Here's how the part is built. I have some questions about the finished solid (model axes, mm). A direction names the side the tool comes from. Round coordinates to 2 decimals unless told otherwise and drop trailing zeros. Order: outer loops, then holes, each group sorted by start corner. A loop starts at its lowest first (then second) coordinate and runs counter-clockwise, first axis right, second up.
```python
from build123d import *

# Parameters (mm, degrees)
SKETCH1_R           = 10.5
SKETCH1_R_2         = 1.85
BOSS_EXTRUDE1_DEPTH = 6
SKETCH2_R           = 5.25
CUT_EXTRUDE1_DEPTH  = 5
SKETCH3_R           = 2.8
CUT_EXTRUDE2_DEPTH  = 2
SKETCH5_R           = 2.85
SKETCH5_R_2         = 1.85
CUT_EXTRUDE4_DEPTH  = 3


with BuildPart() as part:
    # Sketch1 → Boss-Extrude1 (new body)
    with BuildSketch(Plane.XY):
        Circle(SKETCH1_R)
        with Locations((7, 0)):
            Circle(SKETCH1_R_2, mode=Mode.SUBTRACT)
        with Locations((0, -7)):
            Circle(SKETCH1_R_2, mode=Mode.SUBTRACT)
        with Locations((-7, 0)):
            Circle(SKETCH1_R_2, mode=Mode.SUBTRACT)
        with Locations((0, 7)):
            Circle(SKETCH1_R_2, mode=Mode.SUBTRACT)
    extrude(amount=BOSS_EXTRUDE1_DEPTH)

    # Sketch2 → Cut-Extrude1 (cut)
    with BuildSketch(Plane(origin=(0, 0, 0), x_dir=(-1, 0, 0), z_dir=(0, 0, -1))):
        Circle(SKETCH2_R)
    extrude(amount=-CUT_EXTRUDE1_DEPTH, mode=Mode.SUBTRACT)

    # Sketch3 → Cut-Extrude2 (cut, through all)
    with BuildSketch(Plane(origin=(0, 0, 5), x_dir=(-1, 0, 0), z_dir=(0, 0, -1))):
        Circle(SKETCH3_R)
    extrude(amount=-CUT_EXTRUDE2_DEPTH, mode=Mode.SUBTRACT)

    # Sketch5 → Cut-Extrude4 (cut)
    with BuildSketch(Plane(origin=(0, 0, 6), x_dir=(-1, 0, 0), z_dir=(0, 0, -1))):
        with Locations((0, 7)):
            Circle(SKETCH5_R)
        with Locations((0, 7)):
            Circle(SKETCH5_R_2, mode=Mode.SUBTRACT)
        with Locations((7, 0)):
            Circle(SKETCH5_R)
        with Locations((0, -7)):
            Circle(SKETCH5_R)
        with Locations((-7, 0)):
            Circle(SKETCH5_R)
        with Locations((-7, 0)):
            Circle(SKETCH5_R_2, mode=Mode.SUBTRACT)
    extrude(amount=CUT_EXTRUDE4_DEPTH, mode=Mode.SUBTRACT)


solid = part.part
```
1) If we section it at D-D (x = -2.5): Write out the boundary of the cut face in (y, z).
2) I'm going to push flat-ended pins straight in: pin 1 (2.5 mm diameter, centred on x = 0.5, y = -7.5, fed in from +Z); pin 2 (6.5 mm diameter, centred on x = 0, y = -7, fed in from -Z); pin 3 (3 mm diameter, centred on y = -7.5, z = 1.5, fed in from -X); pin 4 (1 mm diameter, centred on x = 6, z = 1, fed in from +Y). Where does each tip first touch, or does it pass through?
3) For faces 4 (the flat face through (9.1, 0, 3)), 5 (the cylindrical face through (-8.85, 0.07, 1.48)), 6 (the cylindrical face through (3.676, 3.748, 1.909)), which set-ups out of +Z, -Z, +X, -X, +Y, -Y let a thin tool reach every point of the face, with its end or its side?
4) If we section it at C-C (z = 1.1): Write out the boundary of the cut face in (x, y).
5) We'd pull the mould along X, two halves only. Please class faces 1 (the cylindrical face through (10, 3.2, 3)), 2 (the flat face through (2.2, -2.2, 6)), 3 (the cylindrical face through (-9.718, 0.856, 4.521)): +X half, -X half, draft (parallel to the pull), parting line (faces both ways), or undercut.
6) If we section it at A-A (x = 0): Write out the boundary of the cut face in (y, z).
7) If we section it at B-B (y = -6.5): Write out the boundary of the cut face in (x, z).
8) I need wall thicknesses on line 1 (Y direction, x = -2.5, z = 4.5); line 2 (Y direction, x = 0, z = 4.1); line 3 (Y direction, x = 0, z = 1.2). Which ranges of each line are inside material? Lowest first, please.
Solutions:
1. outline: (-10.2, 0) - (-4.62, 0) - (-4.62, 5) - (-1.26, 5) - (-1.26, 6) - (-5.63, 6) - (-5.63, 3) - (-8.37, 3) - (-8.37, 6) - (-10.2, 6) - close; (1.26, 5) - (4.62, 5) - (4.62, 0) - (10.2, 0) - (10.2, 6) - (8.37, 6) - (8.37, 3) - (5.63, 3) - (5.63, 6) - (1.26, 6) - close
2. pin 1: stops at z = 3
2. pin 2: stops at z = 0
2. pin 3: stops at x = -8.62
2. pin 4: stops at y = 8.94
3. face 4: +Z
3. face 5: +Z, -Z
3. face 6: -Z
4. outline: circle Ø21 at (0, 0); hole (-5.22, -0.52) arc R5.25 ccw to (-0.52, -5.22) arc R1.85 ccw (long way) to (0.52, -5.22) arc R5.25 ccw to (5.22, -0.52) arc R1.85 ccw (long way) to (5.22, 0.52) arc R5.25 ccw to (0.52, 5.22) arc R1.85 ccw (long way) to (-0.52, 5.22) arc R5.25 ccw to (-5.22, 0.52) arc R1.85 ccw (long way) to start
5. face 1: parting line
5. face 2: draft
5. face 3: undercut
6. outline: (-10.5, 0) - (-8.85, 0) - (-8.85, 3) - (-9.85, 3) - (-9.85, 6) - (-10.5, 6) - close; (-4.15, 5) - (-2.8, 5) - (-2.8, 6) - (-4.15, 6) - close; (2.8, 5) - (4.15, 5) - (4.15, 6) - (2.8, 6) - close; (8.85, 0) - (10.5, 0) - (10.5, 6) - (9.85, 6) - (9.85, 3) - (8.85, 3) - close
7. outline: (-8.25, 0) - (-1.78, 0) - (-1.78, 3) - (-2.81, 3) - (-2.81, 6) - (-8.25, 6) - close; (1.78, 0) - (8.25, 0) - (8.25, 6) - (2.81, 6) - (2.81, 3) - (1.78, 3) - close
8. line 1: y = -10.2 to -8.37, -5.63 to -4.62, 4.62 to 5.63, 8.37 to 10.2
8. line 2: y = -10.5 to -9.85, 9.85 to 10.5
8. line 3: y = -10.5 to -8.85, 8.85 to 10.5
